from build123d import *

# Parameters (mm, degrees)
BASE_DEPTH              = 3
CONG_1_R                = 3
ENL_V_MAT_EXTRU_1_DEPTH = 4
CONG_2_R                = 3
ESQUISSE26_R            = 2
ENL_V_MAT_EXTRU_2_DEPTH = 4
ESQUISSE27_R            = 2
ENL_V_MAT_EXTRU_3_DEPTH = 4
ESQUISSE28_R            = 1.5
ENL_V_MAT_EXTRU_4_DEPTH = 4
ESQUISSE29_R            = 2
ENL_V_MAT_EXTRU_5_DEPTH = 4
ESQUISSE30_R            = 2
ENL_V_MAT_EXTRU_6_DEPTH = 4
ENL_V_MAT_EXTRU_7_DEPTH = 4


with BuildPart() as part:
    # Esquisse1 → Base (new body)
    with BuildSketch(Plane.XY):
        Polygon((0, 0), (-200, 0), (-224.748737342, 24.748737342), (-224.748737342, 284.748737342), (-200, 309.497474683), (0, 309.497474683), (24.748737342, 284.748737342), (24.748737342, 24.748737342), align=None)
    extrude(amount=BASE_DEPTH)

    # Congé1
    cong_1_edges = [part.edges().sort_by_distance(p)[0] for p in [
        (0, 0, 1.5),
        (-200, 0, 1.5),
        (-224.748737342, 24.748737342, 1.5),
        (-224.748737342, 284.748737342, 1.5),
        (-200, 309.497474683, 1.5),
        (0, 309.497474683, 1.5),
        (24.748737342, 284.748737342, 1.5),
        (24.748737342, 24.748737342, 1.5),
    ]]
    fillet(cong_1_edges, radius=CONG_1_R)

    # Esquisse25 → Enlèv. mat.-Extru.1 (cut, through all)
    with BuildSketch(Plane(origin=(0, 0, 0), x_dir=(-1, 0, 0), z_dir=(0, 0, -1))):
        Polygon((-24.748737342, 33), (-24.748737342, 0), (45, 0), (155, 0), (224.748737342, 0), (224.748737342, 33), (224.748737342, 276.497474683), (224.748737342, 309.497474683), (155, 309.497474683), (45, 309.497474683), (-24.748737342, 309.497474683), (-24.748737342, 276.497474683), align=None)
        Polygon((-21.748737342, 33), (45, 33), (45, 3), (155, 3), (155, 33), (221.748737342, 33), (221.748737342, 276.497474683), (155, 276.497474683), (155, 306.497474683), (45, 306.497474683), (45, 276.497474683), (-21.748737342, 276.497474683), align=None, mode=Mode.SUBTRACT)
    extrude(amount=-ENL_V_MAT_EXTRU_1_DEPTH, mode=Mode.SUBTRACT)

    # Congé2
    cong_2_edges = [part.edges().sort_by_distance(p)[0] for p in [
        (21.748737342, 33, 1.5),
        (21.748737342, 276.497474683, 1.5),
        (-45, 306.497474683, 1.5),
        (-155, 306.497474683, 1.5),
        (-221.748737342, 276.497474683, 1.5),
        (-221.748737342, 33, 1.5),
        (-155, 3, 1.5),
        (-45, 3, 1.5),
    ]]
    fillet(cong_2_edges, radius=CONG_2_R)

    # Esquisse26 → Enlèv. mat.-Extru.2 (cut, through all)
    with BuildSketch(Plane(origin=(0, 0, 0), x_dir=(-1, 0, 0), z_dir=(0, 0, -1))):
        with Locations((191.748737342, 189.748737342)):
            Circle(ESQUISSE26_R)
        with Locations((191.748737342, 219.748737342)):
            Circle(ESQUISSE26_R)
        with Locations((191.748737342, 89.748737342)):
            Circle(ESQUISSE26_R)
        with Locations((191.748737342, 119.748737342)):
            Circle(ESQUISSE26_R)
    extrude(amount=-ENL_V_MAT_EXTRU_2_DEPTH, mode=Mode.SUBTRACT)

    # Esquisse27 → Enlèv. mat.-Extru.3 (cut, through all)
    with BuildSketch(Plane(origin=(0, 0, 0), x_dir=(-1, 0, 0), z_dir=(0, 0, -1))):
        with Locations((97.251262658, 53)):
            Circle(ESQUISSE27_R)
        with Locations((18.251262658, 53)):
            Circle(ESQUISSE27_R)
    extrude(amount=-ENL_V_MAT_EXTRU_3_DEPTH, mode=Mode.SUBTRACT)

    # Esquisse28 → Enlèv. mat.-Extru.4 (cut, through all)
    with BuildSketch(Plane(origin=(0, 0, 0), x_dir=(-1, 0, 0), z_dir=(0, 0, -1))):
        with Locations((156.748737342, 195.986237342)):
            Circle(ESQUISSE28_R)
        with Locations((92.998737342, 195.986237342)):
            Circle(ESQUISSE28_R)
        with Locations((156.748737342, 113.511237342)):
            Circle(ESQUISSE28_R)
    extrude(amount=-ENL_V_MAT_EXTRU_4_DEPTH, mode=Mode.SUBTRACT)

    # Esquisse29 → Enlèv. mat.-Extru.5 (cut, through all)
    with BuildSketch(Plane(origin=(0, 0, 0), x_dir=(-1, 0, 0), z_dir=(0, 0, -1))):
        with Locations((156.748737342, 212.497474683)):
            Circle(ESQUISSE29_R)
        with Locations((98.748737342, 212.497474683)):
            Circle(ESQUISSE29_R)
        with Locations((98.748737342, 261.497474683)):
            Circle(ESQUISSE29_R)
        with Locations((156.748737342, 261.497474683)):
            Circle(ESQUISSE29_R)
    extrude(amount=-ENL_V_MAT_EXTRU_5_DEPTH, mode=Mode.SUBTRACT)

    # Esquisse30 → Enlèv. mat.-Extru.6 (cut, through all)
    with BuildSketch(Plane(origin=(0, 0, 0), x_dir=(-1, 0, 0), z_dir=(0, 0, -1))):
        with Locations((64.251262658, 113)):
            Circle(ESQUISSE30_R)
        with Locations((18.251262658, 113)):
            Circle(ESQUISSE30_R)
        with Locations((18.251262658, 168.8)):
            Circle(ESQUISSE30_R)
        with Locations((64.251262658, 168.8)):
            Circle(ESQUISSE30_R)
    extrude(amount=-ENL_V_MAT_EXTRU_6_DEPTH, mode=Mode.SUBTRACT)

    # Esquisse31 → Enlèv. mat.-Extru.7 (cut, through all)
    with BuildSketch(Plane(origin=(0, 0, 0), x_dir=(-1, 0, 0), z_dir=(0, 0, -1))):
        with BuildLine():
            Line((118.251262658, 73), (18.251262658, 73))
            ThreePointArc((18.251262658, 73), (3.251262658, 88), (18.251262658, 103))
            Line((18.251262658, 103), (118.251262658, 103))
            ThreePointArc((118.251262658, 103), (133.251262658, 88), (118.251262658, 73))
        make_face()
    extrude(amount=-ENL_V_MAT_EXTRU_7_DEPTH, mode=Mode.SUBTRACT)


solid = part.part
Can you work these out from the model? Positions are in its coordinate system, mm. A direction names the side the tool comes from. Round coordinates to 2 decimals unless told otherwise and drop trailing zeros. Order: outer loops, then holes, each group sorted by start corner. A loop starts at its lowest first (then second) coordinate and runs counter-clockwise, first axis right, second up. Notation, with made-up numbers: M 57,-20.5 L 87,-20.5 A26 cw 87,13.5 Z; hole C 58.5,-11 d1. An arc over 180 degrees is marked long. Use a Markdown table: item, result.
1) Imagine slicing it at B-B (x = -201). List the corners of the cut face in (y, z) for me.
Geometry says:
| item | result |
|---|---|
| outline | M 33,0 L 276.5,0 L 276.5,3 L 33,3 Z |
2) Imagine slicing it at A-A (x = -107). List the corners of the cut face in (y, z) for me, then the cut area to 3 significant figures.
Geometry says:
| item | result |
|---|---|
| outline | M 3,0 L 73,0 L 73,3 L 3,3 Z; M 103,0 L 306.5,0 L 306.5,3 L 103,3 Z |
| area | 820 mm² |
3) I'm going to push flat-ended pins straight in: P1, Ø5, axis at x = -191.75, y = 119.75, coming from the -Z side; P2, Ø1.5, axis at y = 25.5, z = 2, coming from the -X side; P3, Ø3.5, axis at x = -191.75, y = 189.75, coming from the +Z side; P4, Ø0.9, axis at y = 20.5, z = 2, coming from the +X side. Where does each tip first touch, or does it pass through?
Geometry says:
| item | result |
|---|---|
| P1 | stops at z = 0 |
| P2 | stops at x = -155 |
| P3 | passes through |
| P4 | stops at x = -45 |
4) If we mould it in two halves opening along Y, with no side actions, what happens to faces 3 (the face through (-98, 157, 0)), 4 (the face through (-3.255, 87.67, 1.479))? For each: +Y half, -Y half, draft (parallel to the pull), parting line (faces both ways), or undercut.
Geometry says:
| item | result |
|---|---|
| face 3 | draft |
| face 4 | undercut |
5) On a 3-axis mill with a long thin cutter (end or side, diameter ignored), from which of +Z, -Z, +X, -X, +Y, -Y can I reach the whole of each face in a straight line? I mean faces 1 (the face through (-98, 157, 3)), 2 (the face through (-133.248, 88.33, 1.479)). Say none if no direction works.
Geometry says:
| item | result |
|---|---|
| face 1 | +Z, +X, -X, +Y, -Y |
| face 2 | +Z, -Z |
6) If I drill on line 1 along X through (y, z) = (212, 2.7); line 2 along X through (y, z) = (212.5, 1.15); line 3 along Y through (x, z) = (-85, 2.75), over which ranges is the centre line in solid material (lowest first)?
Geometry says:
| item | result |
|---|---|
| line 1 | x = -221.75 to -158.69, -154.81 to -100.69, -96.81 to 21.75 |
| line 2 | x = -221.75 to -158.75, -154.75 to -100.75, -96.75 to 21.75 |
| line 3 | y = 3 to 73, 103 to 306.5 |
7) Imagine slicing it at C-C (z = 1.7). Give the number of separate pieces and of enclosed holes in the cut face, then the cut area to 3 significant figures.
Geometry says:
| item | result |
|---|---|
| separate pieces | 1 |
| enclosed holes | 18 |
| area | 62,000 mm² |
